from build123d import *

# Parameters (mm, degrees)
PAD_DEPTH    = 14
SKETCH001_W  = 4.2
SKETCH001_H  = 10.937521
POCKET_DEPTH = 28.5


with BuildPart() as part:
    # Sketch → Pad (new body)
    with BuildSketch(Plane.XZ):
        Polygon((0, 30), (14.2, 30), (14.2, 23), (7.2, 23), (7.2, 0), (5.7, 0), (1.5, 0), (0, 0), align=None)
    extrude(amount=PAD_DEPTH)

    # Sketch001 → Pocket (cut)
    with BuildSketch(Plane(origin=(0, 0, 0), x_dir=(1, 0, 0), z_dir=(0, 0, -1))):
        with Locations((3.6, 7.031239)):
            Rectangle(SKETCH001_W, SKETCH001_H)
    extrude(amount=-POCKET_DEPTH, mode=Mode.SUBTRACT)


solid = part.part
Source: CAD feature listing. Evaluate the final solid. Frame: model axes, mm. A direction names the side the tool comes from. Round coordinates to 2 decimals unless told otherwise and drop trailing zeros. Loops run counter-clockwise (first coordinate to the right, second up) from the corner with the lowest first, then second, coordinate; pieces in that order, holes last. Notation, with made-up numbers: (-28, 85) -> (-24, 85) arc R14 cw to (-24, 100) -> close; hole circle Ø11 at (46, 31). An arc over 180 degrees is marked (long way). Answer as a JSON object with one key per item and string values. Group by question number.
Q1. Section query A-A (z = 5.5). Output: boundary loops of the cut face in (x, y), plus the area to 3 significant figures.
Q2. Section query D-D (z = 26). Output: boundary loops of the cut face in (x, y).
Q3. Access query for faces 1 (the flat face through (11, -7, 23)), 2 (the flat face through (6, -14, 19)), 3 (the flat face through (4, -1.562, 14)). Directions: +Z, -Z, +X, -X, +Y, -Y. A direction counts if a zero-diameter tool reaches every point of the face in a straight line with its end or side. Return the directions, or none.
Q4. Section query C-C (x = 2). Output: boundary loops of the cut face in (y, z).
Q5. Section query B-B (y = -9). Output: boundary loops of the cut face in (x, z).
Q6. Mould query, pull axis X, two halves, no side actions, for faces 4 (the flat face through (14.2, -7, 27)), 5 (the flat face through (7, -7, 30)), 6 (the flat face through (4, -7, 28.5)). Classes: pulls with the +X half, pulls with the -X half, needs draft (parallel to the pull), parting line crosses it, or undercut.
Q7. Ray query, line 1 (X direction, y = -4, z = 24); line 2 (X direction, y = -6, z = 7.5); line 3 (Y direction, x = 3, z = 3.5). Return the intervals inside material, ascending. Write a range as from..to.
Q8. Contact query for flat-ended pins moving along their axis: P1, Ø3.5, axis at y = -5.5, z = 11.5, coming from the +X side; P2, Ø5.5, axis at x = 10, y = -9, coming from the -Z side. Output: stop coordinate, or through.
Completed:
{
 "1": {"outline": "(0, -14) -> (7.2, -14) -> (7.2, 0) -> (0, 0) -> close; hole (1.5, -12.5) -> (5.7, -12.5) -> (5.7, -1.56) -> (1.5, -1.56) -> close", "area": "54.9 mm²"},
 "2": {"outline": "(0, -14) -> (14.2, -14) -> (14.2, 0) -> (0, 0) -> close; hole (1.5, -12.5) -> (5.7, -12.5) -> (5.7, -1.56) -> (1.5, -1.56) -> close"},
 "3": {"face 1": "-Z, +X, +Y, -Y", "face 2": "+Z, -Z, +X, -X, -Y", "face 3": "-Z"},
 "4": {"outline": "(-14, 0) -> (-12.5, 0) -> (-12.5, 28.5) -> (-1.56, 28.5) -> (-1.56, 0) -> (0, 0) -> (0, 30) -> (-14, 30) -> close"},
 "5": {"outline": "(0, 0) -> (1.5, 0) -> (1.5, 28.5) -> (5.7, 28.5) -> (5.7, 0) -> (7.2, 0) -> (7.2, 23) -> (14.2, 23) -> (14.2, 30) -> (0, 30) -> close"},
 "6": {"face 4": "pulls with the +X half", "face 5": "needs draft", "face 6": "undercut"},
 "7": {"line 1": "0..1.5, 5.7..14.2", "line 2": "0..1.5, 5.7..7.2", "line 3": "-14..-12.5, -1.56..0"},
 "8": {"P1": "x = 7.2", "P2": "z = 23"}
}
